Input: dimensioned drawing with shaded views. Units: mm. Origin: part minimum x, y, z. A direction names the side the tool comes from. Round coordinates to 2 decimals unless told otherwise and drop trailing zeros. Loops run counter-clockwise (first coordinate to the right, second up) from the corner with the lowest first, then second, coordinate; pieces in that order, holes last.
Item 1: Section query A-A on z = 18. Return loops of the section in (x, y), then the cut area to 3 significant figures.
Item 2: Access query for the marked faces 1 and 2. Directions: +Z, -Z, +X, -X, +Y, -Y. A direction counts if a zero-diameter tool reaches every point of the face in a straight line with its end or side. Return the directions, or none.
Item 3: First-contact query: P1, Ø8, axis at x = 32, z = 2, coming from the +Y side; P2, Ø3, axis at x = 14, y = 10.5, coming from the -Z side (1 decimal); P3, Ø10, axis at x = 17.5, y = 9, coming from the -Z side. Flat tips, straight axial feed; report the tip coordinate or a pass-through.
Item 4: Pull-direction query (X, two-part tool) for the marked faces 3, 4 and 5; classes: released by +X, released by -X, zero draft, split by the parting line, or undercut.
Item 5: Section query C-C on x = 14.5. Return loops of the section in (y, z) (1 decimal).
Item 6: Section query B-B on y = 8.75. Return loops of the section in (x, z).
Item 7: Ray query, L1, parallel to X at y = 13.5, z = 16.75; L2, parallel to Y at x = 11, z = 1.75 (1 decimal); L3, parallel to Z at x = 30.5, y = 6 (1 decimal). Return the intervals inside material, ascending.
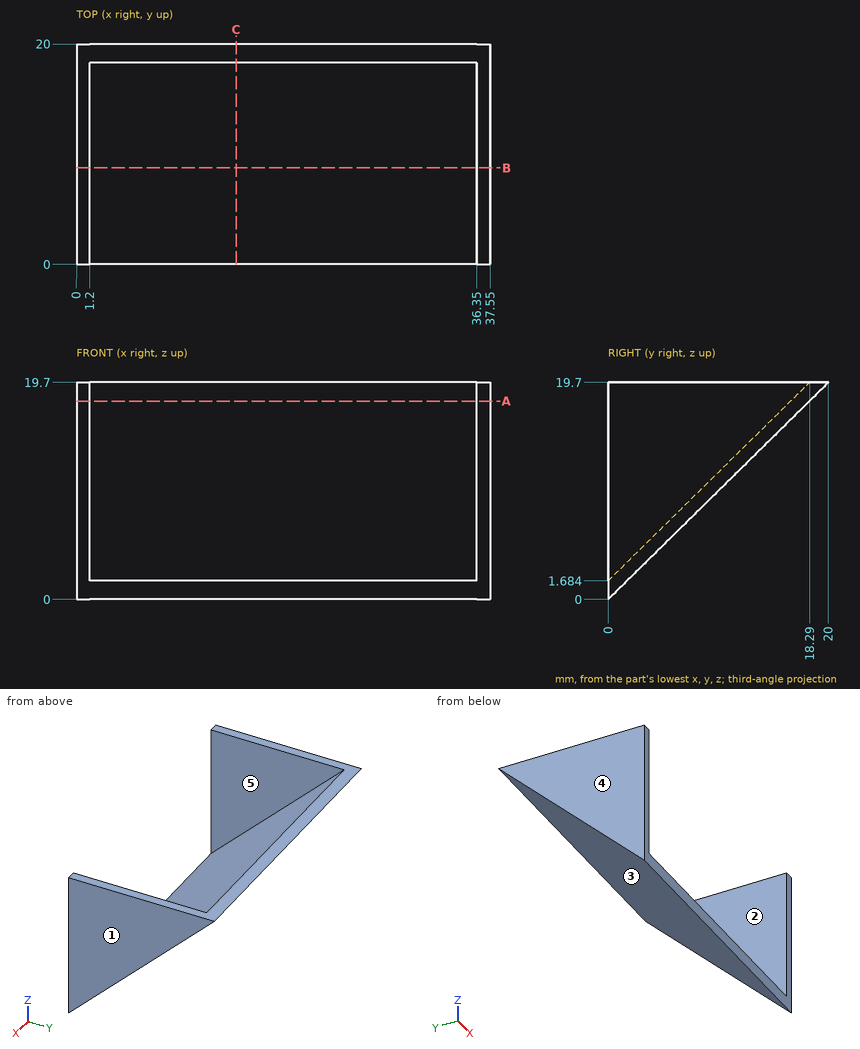
Data:
1. outline: (0, 0) - (1.2, 0) - (1.2, 16.56) - (36.35, 16.56) - (36.35, 0) - (37.55, 0) - (37.55, 18.27) - (0, 18.27) - close
1. area: 104 mm2
2. face 1: +Z, -Z, +X, +Y, -Y
2. face 2: +Z, -Y
3. P1: stops at y = 6.09
3. P2: stops at z = 8.9
3. P3: stops at z = 3.94
4. face 3: zero draft
4. face 4: released by -X
4. face 5: undercut
5. outline: (0, 0) - (20, 19.7) - (18.3, 19.7) - (0, 1.7) - close
6. outline: (0, 8.62) - (37.55, 8.62) - (37.55, 19.7) - (36.35, 19.7) - (36.35, 10.3) - (1.2, 10.3) - (1.2, 19.7) - (0, 19.7) - close
7. L1: x = 0 to 1.2, 36.35 to 37.55
7. L2: y = 0.1 to 1.8
7. L3: z = 5.9 to 7.6
